Input: part model. Units: mm. Frame: model coordinates. A direction names the side the tool comes from. Coordinates: 2 decimals unless noted, no trailing zeros. Order: outer loops, then holes, each group sorted by start corner. A loop starts at its lowest first (then second) coordinate and runs counter-clockwise, first axis right, second up. Notation, with made-up numbers: (63, 84.5) -> (99, 84.5) arc R13 cw to (99, 109.5) -> close; hole circle Ø7 at (88, -31). An arc over 180 degrees is marked (long way). Use one line per item in the form item = value. Start each with the question number.
1) Ray query, line 1 along X through (y, z) = (-117, 5.75); line 2 along X through (y, z) = (-1.5, 2.25); line 3 along Y through (x, z) = (12.5, 0.9). Return the intervals inside material, ascending.
2) Section query C-C on x = 9.5. Output: boundary loops of the cut face in (y, z), then the cut area to 3 significant figures.
3) Section query A-A on x = -15.5. Output: boundary loops of the cut face in (y, z), then the cut area to 3 significant figures.
4) Access query for faces 1 (the flat face through (0, -59, 6)), 2 (the flat face through (-22.5, 0, 3)), 3 (the flat face through (-12, -130, 3)). Directions: +Z, -Z, +X, -X, +Y, -Y. A direction counts if a zero-diameter tool reaches every point of the face in a straight line with its end or side. Return the directions, or none.
5) Draft query along X for faces 4 (the flat face through (-28.5, -62, 3)), 5 (the flat face through (0, 14.5, 3)), 6 (the flat face through (-11.09, 6.28, 2.96)). Return one class per face: pulls with the +X half, pulls with the -X half, needs draft (parallel to the pull), parting line crosses it, or undercut.
6) Section query B-B on z = 1.25. Output: boundary loops of the cut face in (x, y), then the cut area to 3 significant figures.
from build123d import *

# Parameters (mm, degrees)
PAD_DEPTH = 6


with BuildPart() as part:
    # Sketch → Pad (new body)
    with BuildSketch(Plane.XY):
        with BuildLine():
            ThreePointArc((12, -125.5), (0, -113.5), (-12, -125.5))
            Line((-12, -125.5), (-12, -135.5))
            Line((-12, -135.5), (-28.5, -135.5))
            Line((-28.5, -135.5), (-28.5, 14.5))
            Line((-28.5, 14.5), (28.5, 14.5))
            Line((28.5, 14.5), (28.5, -135.5))
            Line((28.5, -135.5), (12, -135.5))
            Line((12, -135.5), (12, -125.5))
        make_face()
        Polygon((0, 8.5), (-22.5, 4), (-22.5, -4), (0, -8.5), (22.5, -4), (22.5, 4), align=None, mode=Mode.SUBTRACT)
    extrude(amount=PAD_DEPTH)


solid = part.part
Answers below:
q1.line_1 = -28.5 to -8.47, 8.47 to 28.5
q1.line_2 = -28.5 to -22.5, 22.5 to 28.5
q1.line_3 = -135.5 to -6, 6 to 14.5
q2.outline = (-118.17, 0) -> (-6.6, 0) -> (-6.6, 6) -> (-118.17, 6) -> close; (6.6, 0) -> (14.5, 0) -> (14.5, 6) -> (6.6, 6) -> close
q2.area = 717 mm^2
q3.outline = (-135.5, 0) -> (-5.4, 0) -> (-5.4, 6) -> (-135.5, 6) -> close; (5.4, 0) -> (14.5, 0) -> (14.5, 6) -> (5.4, 6) -> close
q3.area = 835 mm^2
q4.face_1 = +Z, +X, -X, +Y, -Y
q4.face_2 = +Z, -Z
q4.face_3 = +Z, -Z, -Y
q5.face_4 = pulls with the -X half
q5.face_5 = needs draft
q5.face_6 = undercut
q6.outline = (-28.5, -135.5) -> (-12, -135.5) -> (-12, -125.5) arc R12 cw to (12, -125.5) -> (12, -135.5) -> (28.5, -135.5) -> (28.5, 14.5) -> (-28.5, 14.5) -> close; hole (-22.5, -4) -> (0, -8.5) -> (22.5, -4) -> (22.5, 4) -> (0, 8.5) -> (-22.5, 4) -> close
q6.area = 7,520 mm^2
